Autodesk Inventor part; units mm, degrees
ref_plane "YZ Plane" through (0, 0, 0) normal (1, 0, 0) x (0, 1, 0)
ref_plane "XZ Plane" through (0, 0, 0) normal (0, 1, 0) x (-1, 0, 0)
ref_plane "XY Plane" through (0, 0, 0) normal (0, 0, 1) x (1, 0, 0)
sketch "Sketch1" plane through (0, 0, 0) normal (1, 0, 0) x (0, 1, 0)
  line L0 (0, 0) -> (1828.8, 0)
  line L1 (1828.8, 0) -> (1828.8, -76.2)
  line L2 (1828.8, -76.2) -> (0, -76.2)
  line L3 (0, -76.2) -> (0, 0)
  dimension "d0" = 1828.8
  dimension "d1" = 76.2
extrude "Extrusion1" add sketch "Sketch1" along normal blind 76.2
sketch "Sketch2" plane through (76.2, 0, 0) normal (1, 0, 0) x (0, 0, -1)
  circle A0 centre (38.1, 101.6) radius 25.4
  circle A1 centre (38.1, 203.2) radius 25.4
  circle A2 centre (38.1, 304.8) radius 25.4
  circle A3 centre (38.1, 406.4) radius 25.4
  circle A4 centre (38.1, 508) radius 25.4
  circle A5 centre (38.1, 609.6) radius 25.4
  circle A6 centre (38.1, 711.2) radius 25.4
  circle A7 centre (38.1, 812.8) radius 25.4
  circle A8 centre (38.1, 914.4) radius 25.4
  circle A9 centre (38.1, 1016) radius 25.4
  circle A10 centre (38.1, 1117.6) radius 25.4
  circle A11 centre (38.1, 1219.2) radius 25.4
  circle A12 centre (38.1, 1320.8) radius 25.4
  circle A13 centre (38.1, 1422.4) radius 25.4
  circle A14 centre (38.1, 1524) radius 25.4
  circle A15 centre (38.1, 1625.6) radius 25.4
  circle A16 centre (38.1, 1727.2) radius 25.4
  point P0 (0, 0)
  dimension "d4" = 50.8
  dimension "d5" = 50.8
  dimension "d6" = 50.8
  dimension "d7" = 50.8
  dimension "d8" = 50.8
  dimension "d9" = 50.8
  dimension "d10" = 50.8
  dimension "d11" = 50.8
  dimension "d12" = 50.8
  dimension "d13" = 50.8
  dimension "d14" = 50.8
  dimension "d15" = 50.8
  dimension "d16" = 50.8
  dimension "d17" = 50.8
  dimension "d18" = 50.8
  dimension "d19" = 50.8
  dimension "d20" = 50.8
extrude "Extrusion2" cut sketch "Sketch2" against normal blind 127
sketch "Sketch3" plane through (76.2, 0, 0) normal (1, 0, 0) x (0, 0, -1)
  circle A0 centre (38.1, 38.1) radius 38.1
  circle A1 centre (38.1, 1790.7) radius 38.1
  line L0 (76.2, 1828.8) -> (0, 1828.8)
  line L1 (0, 0) -> (0, 1828.8)
  line L2 (0, 38.1) -> (0, 1790.7)
  line L3 (76.2, 1828.8) -> (76.2, 0)
  line L4 (76.2, 1790.7) -> (76.2, 38.1)
  line L5 (0, 38.1) -> (0, 0)
  line L6 (0, 0) -> (76.2, 0)
  line L7 (76.2, 0) -> (76.2, 38.1)
  circle A2 centre (38.1, 1727.2) radius 25.4
  circle A3 centre (38.1, 1752.6) radius 38.1
  line L8 (0, 1752.6) -> (0, 1738.3207)
  line L9 (76.2, 1752.6) -> (76.2, 1722.009)
  circle A4 centre (38.1, 609.6) radius 25.4
  circle A5 centre (38.1, 584.2) radius 38.1
  line L10 (0, 584.2) -> (0, 799.9293)
  line L11 (76.2, 799.9293) -> (76.2, 584.2)
extrude "Extrusion3" cut sketch "Sketch3" against normal blind 76.2 contours A5 A4 L1 A3 A2 L3 | A5 A4 | A5 A4 | A4 A5 | A3 A2 A1 | A3 A1 A2 | A1 A3 | A3 A2 | A2 A3 keep common part picked at (40.7405, 1765.5775)
properties part number "pole_2"
Geometry check sheet. Reference: the model listing, model coordinates, mm. Coordinates: 2 decimals unless noted, no trailing zeros. Write each loop counter-clockwise with the first axis right and the second up, starting at its lowest first coordinate (ties: lowest second). Pieces come first, ordered by that corner, then holes. Notation, with made-up numbers: (58.25, 85) -> (113.25, 85) arc R16 ccw to (113.25, 94) -> close; hole circle Ø2 at (-32.75, 54). An arc over 180 degrees is marked (long way). One line per question, with ' | ' between items.
1. Thickness scan on probe 1 along Z at (x, y) = (42, 711); probe 2 along Z at (x, y) = (23, 1642.5); probe 3 along Y at (x, z) = (6, -5.5). Record the ranges inside material, lowest first. Write a range as from..to.
Answers:
probe 1: z = -76.2..-63.5, -12.7..0 | probe 2: z = -76.2..-57.06, -19.14..0 | probe 3: y = 564.48..1772.32
2. Cross-section at B-B on y = 1524. Record the cut outline in (x, z).
Answers:
outline: (0, -76.2) -> (76.2, -76.2) -> (76.2, -63.5) -> (0, -63.5) -> close; (0, -12.7) -> (76.2, -12.7) -> (76.2, 0) -> (0, 0) -> close
3. Draft check along Z on faces 1 (the cylindrical face through (38.633, 1702.404, -32.594)), 2 (the cylindrical face through (38.63, 1790.69, -38.94)), 3 (the flat face through (76.2, 1160, -38)). Enter one of: +Z half, -Z half, draft (parallel to the pull), parting line (faces both ways), or undercut.
Answers:
face 1: undercut | face 2: parting line | face 3: draft
4. Cross-section at A-A on x = 42.5. State how many separate pieces and enclosed holes the cut face has, and give its area (3 significant figures).
Answers:
separate pieces: 1 | enclosed holes: 12 | area: 69,300 mm²
5. Depth check by flat-ended pin: pin 1 Ø1.5 at (x, z) = (18, -16) entering from +Y; pin 2 Ø6 at (x, y) = (62.5, 765.5) entering from +Z; pin 3 Ø10 at (x, z) = (64.5, -7.5) entering from +Y; pin 4 Ø2 at (x, z) = (58, -66.5) entering from -Y. Enter the tip coordinate at first touch or a pass-through.
Answers:
pin 1: stops at y = 1784.16 | pin 2: stops at z = 0 | pin 3: stops at y = 1780.82 | pin 4: stops at y = 557.73
